Here's how the part is built. I have some questions about the finished solid (model axes, mm). Face numbers are marked on the shaded views. A direction names the side the tool comes from. Give positions to 0.01 mm unless a question says otherwise; leave off trailing zeros. Loops run counter-clockwise (first coordinate to the right, second up) from the corner with the lowest first, then second, coordinate; pieces in that order, holes last.
Q1. If we section it at C-C (y = 9.5): Please give me the cut outline in (x, z), plus the area to 3 significant figures.
Q2. For the marked faces 1, 2 and 3, which set-ups out of +Z, -Z, +X, -X, +Y, -Y let a thin tool reach every point of the face, with its end or its side?
Q3. I need wall thicknesses on line 1 (X direction, y = 56, z = 15); line 2 (Z direction, x = 23.5, y = 3.5); line 3 (X direction, y = 27, z = 20.5). Which ranges of each line are inside material? Lowest first, please.
Q4. If we section it at A-A (z = 0): Please give me the cut outline in (x, y), plus the area to 3 significant figures.
Q5. We'd pull the mould along X, two halves only. Please class the marked faces 4, 5, 6 and 7: +X half, -X half, draft (parallel to the pull), parting line (faces both ways), or undercut.
Q6. Will these pins go through, and if not, where does the flat tip stop? P1, Ø22, axis at x = 22, z = -0.5, coming from the +Y side; P2, Ø1.5, axis at y = 14, z = 0.5, coming from the +X side; P3, Ø13, axis at y = 32.5, z = 13.5, coming from the +X side; P4, Ø1.5, axis at x = -20, z = 17.5, coming from the -Y side.
Q7. If we section it at B-B (x = 33): Please give me the cut outline in (y, z), plus the area to 3 significant figures.
Q8. If we section it at D-D (x = -35): Please give me the cut outline in (y, z).
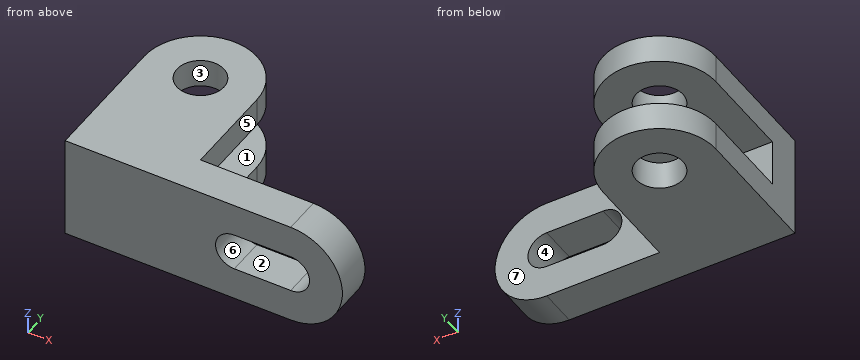
from build123d import *

# Parameters (mm, degrees)
SKETCH1_R           = 22
BOSS_EXTRUDE1_DEPTH = 16
CUT_EXTRUDE2_DEPTH  = 16
BOSS_EXTRUDE2_DEPTH = 12


with BuildPart() as part:
    # Sketch1 → Boss-Extrude1 (new body)
    with BuildSketch(Plane(origin=(0, 0, 0), x_dir=(1, 0, 0), z_dir=(0, 1, 0))):
        with BuildLine():
            Line((37.000000064, 22), (-59, 22))
            Line((-59, 22), (-59, -22))
            Line((-59, -22), (37, -22))
            ThreePointArc((37, -22), (15, 3.2e-08), (37.000000064, 22))
        make_face()
        with Locations((37, 0)):
            Circle(SKETCH1_R)
    extrude(amount=BOSS_EXTRUDE1_DEPTH)

    # Sketch5 → Cut-Extrude2 (cut)
    with BuildSketch(Plane(origin=(0, 16, 0), x_dir=(1, 0, 0), z_dir=(0, 1, 0))):
        with BuildLine():
            Line((37, -8), (13, -8))
            ThreePointArc((13, -8), (5, 0), (13, 8))
            Line((13, 8), (37, 8))
            ThreePointArc((37, 8), (45, 0), (37, -8))
        make_face()
    extrude(amount=-CUT_EXTRUDE2_DEPTH, mode=Mode.SUBTRACT)

    # Sketch6 → Boss-Extrude2 (add)
    with BuildSketch(Plane.XY.offset(22)):
        with BuildLine():
            Line((-59, 56), (-59, 16))
            Line((-59, 16), (-11, 16))
            Line((-11, 16), (-11, 56))
            ThreePointArc((-11, 56), (-35, 32), (-59, 56))
        make_face()
        with BuildLine():
            ThreePointArc((-11, 56), (-35, 80), (-59, 56))
            Line((-59, 56), (-45, 56))
            ThreePointArc((-45, 56), (-35, 66), (-25, 56))
            Line((-25, 56), (-11, 56))
        make_face()
        with BuildLine():
            Line((-45, 56), (-59, 56))
            ThreePointArc((-59, 56), (-35, 32), (-11, 56))
            Line((-11, 56), (-25, 56))
            ThreePointArc((-25, 56), (-35, 46), (-45, 56))
        make_face()
    boss_extrude2 = extrude(amount=-BOSS_EXTRUDE2_DEPTH)

    # Mirror1: Boss-Extrude2 across plane
    add(boss_extrude2.mirror(Plane.XY))


solid = part.part
Check sheet entries:
1. outline: (-59, -22) - (37, -22) arc R22 ccw to (37, 22) - (-59, 22) - close; hole (13, -8) - (37, -8) arc R8 ccw to (37, 8) - (13, 8) arc R8 ccw to start
1. area: 4,400 mm2
2. face 1: +X, -X, +Y
2. face 2: +Y, -Y
2. face 3: +Z, -Z
3. line 1: x = -59 to -45, -25 to -11
3. line 2: z = -22 to -8, 8 to 22
3. line 3: x = -59 to -11
4. outline: (-59, 0) - (5, 0) - (5, 16) - (-59, 16) - close; (45, 0) - (59, 0) - (59, 16) - (45, 16) - close
4. area: 1,250 mm2
5. face 4: undercut
5. face 5: +X half
5. face 6: undercut
5. face 7: draft
6. P1: stops at y = 16
6. P2: stops at x = 59
6. P3: stops at x = -11
6. P4: stops at y = 0
7. outline: (0, -22) - (16, -22) - (16, -8) - (0, -8) - close; (0, 8) - (16, 8) - (16, 22) - (0, 22) - close
7. area: 448 mm2
8. outline: (0, -22) - (46, -22) - (46, -10) - (16, -10) - (16, 10) - (46, 10) - (46, 22) - (0, 22) - close; (66, -22) - (80, -22) - (80, -10) - (66, -10) - close; (66, 10) - (80, 10) - (80, 22) - (66, 22) - close
